from build123d import *

# Parameters (mm, degrees)
SKETCH_1_R               = 20
EXTRUDE_1_DEPTH          = 19.5
CUT_EXTRUDE_START        = 4.5
SKETCH_2_OUTSIDE_W       = 53.968
SKETCH_2_OUTSIDE_H       = 53.968
SKETCH_2_OUTSIDE_R       = 17.5
CUT_EXTRUDE_1_DEPTH      = 30.854766773
CUT_EXTRUDE_START_2      = -14.5
SKETCH_3_OUTSIDE_W       = 53.968
SKETCH_3_OUTSIDE_H       = 53.968
SKETCH_3_OUTSIDE_R       = 15.1
CUT_EXTRUDE_2_DEPTH      = 6
SKETCH_4_R               = 1.25
CUT_EXTRUDE_3_DEPTH      = 35.354766773
SKETCH_4_3_R             = 1.6
CUT_EXTRUDE_4_DEPTH      = 35.354766773
SKETCH_4_4_R             = 3.25
CUT_EXTRUDE_5_DEPTH      = 4
PATTERN_CIRCULAR_1_COUNT = 3
CHAMFER_1_SIZE           = 0.5
SKETCH_4_5_R             = 3
SKETCH_4_5_R_2           = 1.25
CUT_EXTRUDE_6_DEPTH      = 4
CHAMFER_2_SIZE           = 0.3


with BuildPart() as part:
    # Sketch 1 → Extrude 1 (new body)
    with BuildSketch(Plane(origin=(0, 0, 0), x_dir=(1, 0, 0), z_dir=(0, 1, 0))):
        with Locations(Location((0, 0, 0), (0, 0, 270))):
            Circle(SKETCH_1_R)
    extrude(amount=EXTRUDE_1_DEPTH)

    # Sketch 2 outside → Cut-Extrude 1 (cut, through all)
    with BuildSketch(Plane(origin=(0, 0, 0), x_dir=(1, 0, 0), z_dir=(0, 1, 0)).offset(CUT_EXTRUDE_START)):
        Rectangle(SKETCH_2_OUTSIDE_W, SKETCH_2_OUTSIDE_H)
        with Locations(Location((0, 0, 0), (0, 0, 270))):
            Circle(SKETCH_2_OUTSIDE_R, mode=Mode.SUBTRACT)
    extrude(amount=CUT_EXTRUDE_1_DEPTH, mode=Mode.SUBTRACT)

    # Sketch 3 outside → Cut-Extrude 2 (cut)
    with BuildSketch(Plane.XZ.offset(CUT_EXTRUDE_START_2)):
        Rectangle(SKETCH_3_OUTSIDE_W, SKETCH_3_OUTSIDE_H)
        with Locations(Location((0, 0, 0), (0, 0, 270))):
            Circle(SKETCH_3_OUTSIDE_R, mode=Mode.SUBTRACT)
    extrude(amount=-CUT_EXTRUDE_2_DEPTH, mode=Mode.SUBTRACT)

    # Sketch 4 → Cut-Extrude 3 (cut, through all)
    with BuildSketch(Plane(origin=(0, 0, 0), x_dir=(1, 0, 0), z_dir=(0, 1, 0))):
        with Locations(Location((0, 0, 0), (0, 0, 270))):
            Circle(SKETCH_4_R)
    extrude(amount=CUT_EXTRUDE_3_DEPTH, mode=Mode.SUBTRACT)

    # Sketch 4_3 → Cut-Extrude 4 (cut, through all)
    with BuildSketch(Plane(origin=(0, 0, 0), x_dir=(1, 0, 0), z_dir=(0, 1, 0))):
        with Locations(Location((0, 12, 0), (0, 0, 270))):
            Circle(SKETCH_4_3_R)
    cut_extrude_4 = extrude(amount=CUT_EXTRUDE_4_DEPTH, mode=Mode.SUBTRACT)

    # Sketch 4_4 → Cut-Extrude 5 (cut)
    with BuildSketch(Plane(origin=(0, 0, 0), x_dir=(1, 0, 0), z_dir=(0, 1, 0))):
        with Locations(Location((0, 12, 0), (0, 0, 270))):
            Circle(SKETCH_4_4_R)
    cut_extrude_5 = extrude(amount=CUT_EXTRUDE_5_DEPTH, mode=Mode.SUBTRACT)

    # Pattern Circular 1: Cut-Extrude 4, Cut-Extrude 5 ×3 about axis
    pattern_circular_1_axis = Axis((0, 0, 0), (0, 1, 0))
    add([cut_extrude_4.rotate(pattern_circular_1_axis, i * 360 / PATTERN_CIRCULAR_1_COUNT) for i in range(1, PATTERN_CIRCULAR_1_COUNT)], mode=Mode.SUBTRACT)
    add([cut_extrude_5.rotate(pattern_circular_1_axis, i * 360 / PATTERN_CIRCULAR_1_COUNT) for i in range(1, PATTERN_CIRCULAR_1_COUNT)], mode=Mode.SUBTRACT)

    # Chamfer 1
    chamfer_1_edges = [part.edges().sort_by_distance(p)[0] for p in [
        (0, 0, -20),
        (0, 14.5, -17.5),
        (0, 19.5, 15.1),
        (0, 4.5, -20),
    ]]
    chamfer(chamfer_1_edges, length=CHAMFER_1_SIZE)

    # Sketch 4_5 → Cut-Extrude 6 (cut)
    with BuildSketch(Plane(origin=(0, 0, 0), x_dir=(1, 0, 0), z_dir=(0, 1, 0))):
        with Locations(Location((0, 0, 0), (0, 0, 270))):
            Circle(SKETCH_4_5_R)
        with Locations(Location((0, 0, 0), (0, 0, 270))):
            Circle(SKETCH_4_5_R_2, mode=Mode.SUBTRACT)
    extrude(amount=CUT_EXTRUDE_6_DEPTH, mode=Mode.SUBTRACT)

    # Chamfer 2
    chamfer_2_edges = [part.edges().sort_by_distance(p)[0] for p in [
        (0, 19.5, -1.25),
        (0, 0, -3),
    ]]
    chamfer(chamfer_2_edges, length=CHAMFER_2_SIZE)


solid = part.part
Read the model definition and answer for the solid it produces. Units are mm, in the model's axes. A direction names the side the tool comes from. Coordinates: 2 decimals unless noted, no trailing zeros. Write each loop counter-clockwise with the first axis right and the second up, starting at its lowest first coordinate (ties: lowest second). Pieces come first, ordered by that corner, then holes. Notation, with made-up numbers: (-12.75, 72.5) - (10.25, 72.5) arc R6 ccw to (10.25, 80.5) - close; hole circle Ø1 at (-13, 38). An arc over 180 degrees is marked (long way). One line per question, with ' | ' between items.
Q1. Consider L1, parallel to Z at x = 0, y = 9.25; L2, parallel to X at y = 12, z = 6; L3, parallel to Y at x = 5, z = 17. Determine where each line is inside the solid, lowest interval first. Write a range as [from, to].
Result set:
L1: [-17.5, -13.6], [-10.4, -1.25], [1.25, 17.5] | L2: [-16.44, -11.99], [-8.79, 8.79], [11.99, 16.44] | L3: [0, 4.5]
Q2. Each of these flat-tipped pins is pushed along its axis until it touches: P1, Ø1, axis at x = -9.5, z = -5.5, coming from the -Y side; P2, Ø1, axis at x = 7.5, y = 2, coming from the -Z side (3 decimals); P3, Ø2, axis at y = 17, z = 13, coming from the +X side; P4, Ø4, axis at x = -13.5, y = 14, coming from the -Z side. Where does it stop, or does it pass through?
Result set:
P1: y = 0 | P2: z = -18.735 | P3: x = 9.17 | P4: z = -13.19
Q3. For faces 5 (the cylindrical face through (-10.648, 9.183, -13.887)), 6 (the cylindrical face through (-11.005, 11.642, 7.478)), 7 (the flat face through (10, 4, 8)), determine the directions among +Z, -Z, +X, -X, +Y, -Y from which every point of the face is accessible in a straight line to the end or side of a thin tool.
Result set:
face 5: +Y | face 6: +Y, -Y | face 7: -Y
Q4. Find section B-B, the plane x = 0. State how many separate pieces and enclosed holes the cut face has, plus the area to 3 significant figures.
Result set:
separate pieces: 3 | enclosed holes: 0 | area: 541 mm^2
Q5. Determine the mould class of faces 1 (the cylindrical face through (11.98, 11.64, 5.79)), 2 (the flat face through (-13, 4.5, -12)), 3 (the cylindrical face through (-19.524, 2.226, -4.336)), 4 (the cylindrical face through (0.9, 2.12, 2.86)) for opening direction X: +X half, -X half, draft (parallel to the pull), parting line (faces both ways), or undercut.
Result set:
face 1: undercut | face 2: draft | face 3: parting line | face 4: undercut
Q6. Find section C-C, the plane y = 2. Write down the section's boundary in (x, z) (3 decimals).
Result set:
outline: circle Ø40 at (0, 0); hole circle Ø6.5 at (-10.392, 6); hole circle Ø6.5 at (0, -12); hole circle Ø6 at (0, 0); hole circle Ø6.5 at (10.392, 6)
